Autodesk Inventor part; units mm, degrees
ref_plane "YZ Plane" through (0, 0, 0) normal (1, 0, 0) x (0, 1, 0)
ref_plane "XZ Plane" through (0, 0, 0) normal (0, 1, 0) x (-1, 0, 0)
ref_plane "XY Plane" through (0, 0, 0) normal (0, 0, 1) x (1, 0, 0)
sketch "Sketch1" plane through (0, 0, 0) normal (0, 1, 0) x (-1, 0, 0)
  line L0 (-149, -224) -> (149, -224)
  line L1 (149, -224) -> (149, 224)
  line L2 (149, 224) -> (-149, 224)
  line L3 (-149, 224) -> (-149, -224)
  line L4 (-149, -224) -> (149, 224) construction
  line L5 (149, -224) -> (-149, 224) construction
  point P0 (0, 0)
  point P1 (132, 210)
  point P2 (-132, -210)
  point P3 (132, -210)
  point P4 (-132, 210)
  dimension "d0" = 298
  dimension "d1" = 448
extrude "Extrusion1" add sketch "Sketch1" along normal blind 3
sketch "Sketch2" plane through (0, 3, 0) normal (0, 1, 0) x (1, 0, 0)
  line L0 (-149, 224) -> (-149, -224)
  line L1 (-149, -224) -> (149, -224)
  line L2 (149, -224) -> (149, 224)
  line L3 (149, 224) -> (-149, 224)
  line L4 (-149, 224) -> (-149, -224)
  line L5 (-149, -224) -> (149, -224)
  line L6 (149, -224) -> (149, 224)
  line L7 (149, 224) -> (-149, 224)
  line L8 (-146, -221) -> (-146, 221)
  line L9 (-146, 221) -> (146, 221)
  line L10 (146, 221) -> (146, -221)
  line L11 (146, -221) -> (-146, -221)
  point P0 (0, 0)
  dimension "d4" = 3
extrude "Extrusion2" add sketch "Sketch2" along normal blind 50 and the other way blind 65
hole "Hole1" at (132, 0, -210) at (132, 0, 210) at (-132, 0, 210) at (-132, 0, -210) direction (0, 1, 0) diameter 5 end through all
sketch "Sketch3" plane through (149, -62, -224) normal (1, 0, 0) x (0, 0, -1)
  line L0 (0, 0) -> (0, 115)
  line L1 (-448, 115) -> (0, 115)
  line L2 (-448, 0) -> (-448, 115)
  line L3 (0, 0) -> (-448, 0)
  point P0 (-224, 62)
sketch "Sketch4" plane through (149, -62, -224) normal (1, 0, 0) x (0, 0, -1)
  line L0 (0, 0) -> (0, 115)
  line L1 (-448, 115) -> (0, 115)
  line L2 (-448, 0) -> (-448, 115)
  line L3 (0, 0) -> (-448, 0)
  point P0 (-224, 62)
sketch "Sketch5" plane through (149, -62, -224) normal (1, 0, 0) x (0, 0, -1)
  line L0 (0, 0) -> (0, 115)
  line L1 (-448, 115) -> (0, 115)
  line L2 (-448, 0) -> (-448, 115)
  line L3 (0, 0) -> (-448, 0)
  line L4 (0, 0) -> (-448, 0)
  point P0 (-224, 62)
  point P1 (-224, 62)
  point P2 (-99, 25)
  dimension "d16" = 99
  dimension "d17" = 25
sketch "Sketch6" plane through (149, -62, -224) normal (1, 0, 0) x (0, 0, -1)
  line L0 (0, 0) -> (-448, 0)
  line L1 (-445, 115) -> (-3, 115)
  line L2 (-224, 115) -> (-224, 0)
  line L3 (-79, 0) -> (-119, 0)
  line L4 (-119, 0) -> (-119, 30)
  line L5 (-99, 50) -> (-99, 50)
  line L6 (-79, 30) -> (-79, 0)
  line L7 (-79, 0) -> (-119, 50) construction
  line L8 (-119, 0) -> (-79, 50) construction
  line L9 (-448, 0) -> (-448, 115)
  arc A0 (-99, 50) -> (-119, 30) centre (-99, 30) ccw
  arc A1 (-79, 30) -> (-99, 50) centre (-99, 30) ccw
  line L10 (-329, 0) -> (-329, 30)
  line L11 (-369, 30) -> (-369, 0)
  line L12 (-369, 0) -> (-329, 50) construction
  line L13 (-329, 0) -> (-369, 50) construction
  arc A2 (-329, 30) -> (-349, 50) centre (-349, 30) ccw
  arc A3 (-349, 50) -> (-369, 30) centre (-349, 30) ccw
  line L14 (-304.3108, 54.0001) -> (-144.3108, 54.0001) construction
  line L15 (-445, 62) -> (-3, 62)
  line L16 (-304.3108, 36.5001) -> (-144.3108, 36.5001)
  line L17 (-144.3108, 71.5001) -> (-304.3108, 71.5001)
  arc A4 (-304.3108, 71.5001) -> (-304.3108, 36.5001) centre (-304.3108, 54.0001) ccw
  arc A5 (-144.3108, 36.5001) -> (-144.3108, 71.5001) centre (-144.3108, 54.0001) ccw
  point P0 (-224, 62)
  point P1 (-99, 25)
  point P2 (-99, 25)
  point P3 (-99, 25)
  point P4 (-119, 0)
  point P5 (-79, 0)
  point P6 (-349, 25)
  point P7 (-349, 25)
  point P8 (-99, 50)
  point P9 (-349, 50)
  point P10 (-329, 0)
  point P11 (-224.3108, 54.0001)
  point P12 (-304.3108, 54.0001)
  dimension "d18" = 40
  dimension "d19" = 50
  dimension "d26" = 20
  dimension "d27" = 20
  dimension "d28" = 99
  dimension "d29" = 25
  dimension "d32" = 35
extrude "Extrusion3" cut sketch "Sketch6" against normal through all contours L0 L4 A0 A1 L6
extrude "Extrusion4" cut sketch "Sketch6" against normal through all contours L0 L11 A3 A2 L10
extrude "Extrusion5" cut sketch "Sketch6" against normal blind 3 contours L16 A4 L15 L2 | L2 L15 A5 L16 | L15 A4 L17 L2 | L2 L17 A5 L15
sketch "Sketch7" plane through (149, -62, -224) normal (1, 0, 0) x (0, 0, -1)
  arc A0 (-144.3108, 36.5001) -> (-144.3108, 71.5001) centre (-144.3108, 54.0001) ccw
  line L0 (-144.3108, 36.5001) -> (-304.3108, 36.5001)
  arc A1 (-304.3108, 71.5001) -> (-304.3108, 36.5001) centre (-304.3108, 54.0001) ccw
  line L1 (-304.3108, 71.5001) -> (-144.3108, 71.5001)
  line L2 (-369, 0) -> (-369, 30)
  arc A2 (-329, 30) -> (-369, 30) centre (-349, 30) ccw
  line L3 (-329, 30) -> (-329, 0)
  line L4 (-119, 0) -> (-329, 0)
  line L5 (-119, 0) -> (-119, 30)
  arc A3 (-79, 30) -> (-119, 30) centre (-99, 30) ccw
  line L6 (-79, 30) -> (-79, 0)
  line L7 (0, 0) -> (-79, 0)
  line L8 (0, 0) -> (0, 115)
  line L9 (-448, 115) -> (0, 115)
  line L10 (-448, 0) -> (-448, 115)
  line L11 (-369, 0) -> (-448, 0)
  point P0 (-224, 62)
ref_plane "Work Plane2" through (0, -62, -224) normal (1, 0, 0) x (0, 0, -1)
sketch "Sketch8" plane through (149, -62, -224) normal (1, 0, 0) x (0, 0, -1)
  arc A0 (-144.3108, 36.5001) -> (-144.3108, 71.5001) centre (-144.3108, 54.0001) ccw
  line L0 (-144.3108, 36.5001) -> (-304.3108, 36.5001)
  arc A1 (-304.3108, 71.5001) -> (-304.3108, 36.5001) centre (-304.3108, 54.0001) ccw
  line L1 (-304.3108, 71.5001) -> (-144.3108, 71.5001)
  line L2 (-369, 0) -> (-369, 30)
  arc A2 (-329, 30) -> (-369, 30) centre (-349, 30) ccw
  line L3 (-329, 30) -> (-329, 0)
  line L4 (-119, 0) -> (-329, 0)
  line L5 (-119, 0) -> (-119, 30)
  arc A3 (-79, 30) -> (-119, 30) centre (-99, 30) ccw
  line L6 (-79, 30) -> (-79, 0)
  line L7 (0, 0) -> (-79, 0)
  line L8 (0, 0) -> (0, 115)
  line L9 (-448, 115) -> (0, 115)
  line L10 (-448, 0) -> (-448, 115)
  line L11 (-369, 0) -> (-448, 0)
  point P0 (-224, 62)
mirror "Mirror1" about plane through (0, -62, -224) normal (1, 0, 0) of "Extrusion5"
properties part number "AMR_Top_Basket"
Read the model definition and answer for the solid it produces. Units are mm, in the model's axes. A direction names the side the tool comes from. Round coordinates to 2 decimals unless told otherwise and drop trailing zeros. Loops run counter-clockwise (first coordinate to the right, second up) from the corner with the lowest first, then second, coordinate; pieces in that order, holes last.
Q1. Each of these flat-tipped pins is pushed along its axis until it touches: pin 1 (12 mm diameter, centred on x = 78, z = -12.5, fed in from +Y); pin 2 (4 mm diameter, centred on x = 47.5, z = 133.5, fed in from -Y); pin 3 (3 mm diameter, centred on x = 132, z = 210, fed in from -Y). Where does it stop, or does it pass through?
Q2. Determine the mould class of faces 1 (the face through (-1, -62, 222)), 2 (the face through (-147.521, -7.615, -97.185)), 3 (the face through (-149, -31, -3)), 4 (the face through (147.521, -8.385, -97.185)) for opening direction Y: released by +Y, released by -Y, zero draft, split by the parting line, or undercut.
Q3. Section A-A on y = 33 is taken. Write down the section's boundary in (x, z), and give its area (3 significant figures).
Q4. Section D-D on z = -125 is taken. Write down the section's boundary in (x, y), and give its area (3 significant figures).
Q5. Consider probe 1 along Z at (x, y) = (132, 2); probe 2 along X at (y, z) = (1.8, -210); probe 3 along Z at (x, y) = (5.5, 8.5). Determine where each line is inside the solid, lowest interval first.
Q6. Section C-C on x = -27.5 is taken. Write down the section's boundary in (y, z), and give its area (3 significant figures).
Q7. Which of the six approach directions +Z, -Z, +X, -X, +Y, -Y give full straight-line access (tool end or side, diameter ignored) to faces 5 (the face through (2, 0, 3)), 6 (the face through (-146, 28, 3)), 7 (the face through (148, -12, 125))?
Q8. Section B-B on z = 15 is taken. Write down the section's boundary in (x, y).
Output:
1. pin 1: stops at y = 3
1. pin 2: stops at y = 0
1. pin 3: passes through
2. face 1: released by -Y
2. face 2: undercut
2. face 3: zero draft
2. face 4: undercut
3. outline: (-149, -224) - (149, -224) - (149, 224) - (-149, 224) - close; hole (-146, -221) - (146, -221) - (146, 221) - (-146, 221) - close
3. area: 4,440 mm2
4. outline: (-149, -12) - (-146, -12) - (-146, 0) - (146, 0) - (146, -12) - (149, -12) - (149, 53) - (146, 53) - (146, 3) - (-146, 3) - (-146, 53) - (-149, 53) - close
4. area: 1,270 mm2
5. probe 1: z = -224 to -212.5, -207.5 to 207.5, 212.5 to 224
5. probe 2: x = -149 to -134.5, -129.5 to 129.5, 134.5 to 149
5. probe 3: z = -224 to -221, 221 to 224
6. outline: (-62, -224) - (53, -224) - (53, -221) - (3, -221) - (3, 221) - (53, 221) - (53, 224) - (-62, 224) - (-62, 221) - (0, 221) - (0, -221) - (-62, -221) - close
6. area: 2,020 mm2
7. face 5: -Y
7. face 6: +Y
7. face 7: +X, -X, -Y
8. outline: (-149, -62) - (-146, -62) - (-146, -25.5) - (-149, -25.5) - close; (-149, 9.5) - (-146, 9.5) - (-146, 53) - (-149, 53) - close; (-146, 0) - (146, 0) - (146, 3) - (-146, 3) - close; (146, -62) - (149, -62) - (149, -25.5) - (146, -25.5) - close; (146, 9.5) - (149, 9.5) - (149, 53) - (146, 53) - close
